Source: CAD feature listing. Evaluate the final solid. Frame: model axes, mm. Face numbers are marked on the shaded views. A direction names the side the tool comes from. Give positions to 0.01 mm unless a question says otherwise; leave off trailing zeros. Write each loop counter-clockwise with the first axis right and the second up, starting at its lowest first coordinate (ties: lowest second). Pieces come first, ordered by that corner, then holes. Notation, with made-up numbers: (45, 50) -> (65, 50) arc R9 cw to (65, 56) -> close; hole circle Ø10 at (39, 45.25). An arc over 180 degrees is marked (long way). Write item = value, one per line.
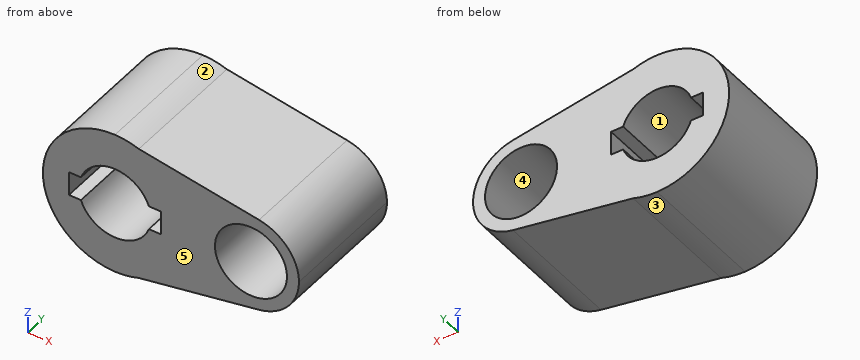
from build123d import *

# Parameters (mm, degrees)
F0_R     = 14.2875
F1_DEPTH = 50.8


with BuildPart() as f1:
    # F0 (on Front) → F1 (new body)
    with BuildSketch(Plane.XZ):
        with BuildLine():
            Line((9.512184, 26.945296), (0, 28.575))
            ThreePointArc((0, 28.575), (-28.575, 0), (0, -28.575))
            Line((0, -28.575), (9.512184, -26.945296))
            ThreePointArc((9.512184, -26.945296), (23.327466, -16.503332), (28.575, 0))
            ThreePointArc((28.575, 0), (23.327466, 16.503332), (9.512184, 26.945296))
        make_face()
        with BuildLine():
            ThreePointArc((-13.470384, 4.7625), (0, 14.2875), (13.470384, 4.7625))
            Line((13.470384, 4.7625), (18.248519, 4.7625))
            Line((18.248519, 4.7625), (18.248519, -4.7625))
            Line((18.248519, -4.7625), (13.470384, -4.7625))
            ThreePointArc((13.470384, -4.7625), (0, -14.2875), (-13.470384, -4.7625))
            Line((-13.470384, -4.7625), (-18.248519, -4.7625))
            Line((-18.248519, -4.7625), (-18.248519, 4.7625))
            Line((-18.248519, 4.7625), (-13.470384, 4.7625))
        make_face(mode=Mode.SUBTRACT)
        with BuildLine():
            ThreePointArc((9.512184, 26.945296), (4.825391, 28.164627), (0, 28.575))
            Line((0, 28.575), (9.512184, 26.945296))
        make_face()
        with BuildLine():
            Line((9.512184, -26.945296), (0, -28.575))
            ThreePointArc((0, -28.575), (4.825391, -28.164627), (9.512184, -26.945296))
        make_face()
        with BuildLine():
            Line((57.191927, 18.776418), (9.512184, 26.945296))
            ThreePointArc((9.512184, 26.945296), (23.327466, 16.503332), (28.575, 0))
            ThreePointArc((28.575, 0), (23.327466, -16.503332), (9.512184, -26.945296))
            Line((9.512184, -26.945296), (57.191927, -18.776418))
            ThreePointArc((57.191927, -18.776418), (34.925, 0), (57.191927, 18.776418))
        make_face()
        with BuildLine():
            ThreePointArc((73.025, 0), (68.538395, 12.280473), (57.191927, 18.776418))
            ThreePointArc((57.191927, 18.776418), (34.925, 0), (57.191927, -18.776418))
            ThreePointArc((57.191927, -18.776418), (68.538395, -12.280473), (73.025, 0))
        make_face()
        with Locations((53.975, 0)):
            Circle(F0_R, mode=Mode.SUBTRACT)
    extrude(amount=F1_DEPTH)


solid = f1.part
(1) Material intervals for line 1 (X direction, y = -7, z = 5); line 2 (X direction, y = -36.5, z = 3); line 3 (Z direction, x = 9.5, y = -21), sorted ascending.
Values follow:
line_1 = -28.13 to -13.38, 13.38 to 40.59, 67.36 to 72.36
line_2 = -28.42 to -18.25, 18.25 to 40.01, 67.94 to 72.79
line_3 = -26.95 to -10.67, 10.67 to 26.95
(2) Section query D-D (z = -23.5). Return loops of the section in (x, y).
Values follow:
outline = (-16.26, -50.8) -> (29.62, -50.8) -> (29.62, 0) -> (-16.26, 0) -> close
(3) Pull-direction query (Z, two-part tool) for the marked faces 3, 4 and 5; classes: pulls with the +Z half, pulls with the -Z half, needs draft (parallel to the pull), parting line crosses it, or undercut.
Values follow:
face_3 = pulls with the -Z half
face_4 = undercut
face_5 = needs draft
(4) Section query B-B (z = -13). Return loops of the section in (x, y).
Values follow:
outline = (-25.45, -50.8) -> (-5.93, -50.8) -> (-5.93, 0) -> (-25.45, 0) -> close; (5.93, -50.8) -> (48.05, -50.8) -> (48.05, 0) -> (5.93, 0) -> close; (59.9, -50.8) -> (67.9, -50.8) -> (67.9, 0) -> (59.9, 0) -> close
(5) Access query for the marked faces 1 and 2. Directions: +Z, -Z, +X, -X, +Y, -Y. A direction counts if a zero-diameter tool reaches every point of the face in a straight line with its end or side. Return the directions, or none.
Values follow:
face_1 = +Y, -Y
face_2 = +Z, +X, +Y, -Y
(6) First-contact query: pin 1 (5.5 mm diameter, centred on x = 15, y = -16, fed in from -Z); pin 2 (4 mm diameter, centred on x = 16, y = -27, fed in from +Z); pin 3 (3 mm diameter, centred on x = 38, z = -18.5, fed in from +Y); pin 4 (4 mm diameter, centred on x = -16, y = -26.5, fed in from -Z). Flat tips, straight axial feed; report the tip coordinate or a pass-through.
Values follow:
pin_1 = -26.48
pin_2 = 26.18
pin_3 = 0
pin_4 = -24.91
(7) Section query C-C (x = 23). Return loops of the section in (y, z), plus the area to 3 significant figures.
Values follow:
outline = (-50.8, -24.63) -> (0, -24.63) -> (0, 24.63) -> (-50.8, 24.63) -> close
area = 2,500 mm2
(8) Section query A-A (y = -44). Give the number of separate pieces and of enclosed holes in the cut face, plus the area to 3 significant figures.
Values follow:
separate_pieces = 1
enclosed_holes = 2
area = 3,080 mm2
